Work out the finished part from the listing and answer in its coordinate system (mm). A direction names the side the tool comes from. Give positions to 0.01 mm unless a question says otherwise; leave off trailing zeros. Loops run counter-clockwise (first coordinate to the right, second up) from the corner with the lowest first, then second, coordinate; pieces in that order, holes last. Notation, with made-up numbers: (55, 64) - (69, 64) arc R13 ccw to (69, 89) - close; hole circle Ø3 at (-4, 0). An arc over 180 degrees is marked (long way). One line per item, written item: value.
from build123d import *

# Parameters (mm, degrees)
SKETCH1_W           = 25.4
SKETCH1_H           = 50.8
SKETCH1_W_2         = 19.05
SKETCH1_H_2         = 44.45
BOSS_EXTRUDE1_DEPTH = 736.6
SKETCH4_R           = 3.175
CUT_EXTRUDE1_DEPTH  = 3.175


with BuildPart() as part:
    # Sketch1 → Boss-Extrude1 (new body)
    with BuildSketch(Plane.XY):
        with Locations((12.7, 25.4)):
            Rectangle(SKETCH1_W, SKETCH1_H)
        with Locations((12.7, 25.4)):
            Rectangle(SKETCH1_W_2, SKETCH1_H_2, mode=Mode.SUBTRACT)
    extrude(amount=BOSS_EXTRUDE1_DEPTH)

    # Sketch4 → Cut-Extrude1 (cut)
    with BuildSketch(Plane.XZ):
        with Locations((12.7, 710.541764528)):
            Circle(SKETCH4_R)
        with Locations((12.7, 725.17)):
            Circle(SKETCH4_R)
        with Locations((12.7, 11.43)):
            Circle(SKETCH4_R)
        with Locations((12.7, 26.058235472)):
            Circle(SKETCH4_R)
    extrude(amount=-CUT_EXTRUDE1_DEPTH, mode=Mode.SUBTRACT)


solid = part.part
1. For faces 1 (the flat face through (13, 50.8, 363)), 2 (the flat face through (3.175, 25, 363)), determine the directions among +Z, -Z, +X, -X, +Y, -Y from which every point of the face is accessible in a straight line to the end or side of a thin tool.
Output:
face 1: +Z, -Z, +X, -X, +Y
face 2: +Z, -Z
2. Section A-A (z = 599) is taken. Write down the section's boundary in (x, y) (3 decimals).
Output:
outline: (0, 0) - (25.4, 0) - (25.4, 50.8) - (0, 50.8) - close; hole (3.175, 3.175) - (22.225, 3.175) - (22.225, 47.625) - (3.175, 47.625) - close
3. Flat-ended cylindrical pins translate along their axes: pin 1 Ø10 at (x, y) = (4.5, 21.5) entering from -Z; pin 2 Ø4 at (x, y) = (19, 15.5) entering from -Z; pin 3 Ø5.5 at (x, z) = (12.7, 11.43) entering from -Y (3 decimals). Find the tip coordinate at first contact, or state that the pin passes through.
Output:
pin 1: stops at z = 0
pin 2: passes through
pin 3: stops at y = 47.625
4. Find the intervals of material crossed by line 1 along Z through (x, y) = (12.7, 1.4) (3 decimals); line 2 along X through (y, z) = (8, 258) (3 decimals); line 3 along Y through (x, z) = (10.75, 615.5) (3 decimals), in increasing order.
Output:
line 1: z = 0 to 8.255, 14.605 to 22.883, 29.233 to 707.367, 713.717 to 721.995, 728.345 to 736.6
line 2: x = 0 to 3.175, 22.225 to 25.4
line 3: y = 0 to 3.175, 47.625 to 50.8
5. Section B-B (y = 16.5) is taken. Write down the section's boundary in (x, z) (3 decimals).
Output:
outline: (0, 0) - (3.175, 0) - (3.175, 736.6) - (0, 736.6) - close; (22.225, 0) - (25.4, 0) - (25.4, 736.6) - (22.225, 736.6) - close
6. The mould has two halves that part along Y. Classify faces 3 (the flat face through (2, 24, 736.6)), 4 (the flat face through (13, 0, 363)), 5 (the flat face through (13, 3.175, 363)), 6 (the flat face through (13, 47.625, 363)): released by +Y, released by -Y, zero draft, split by the parting line, or undercut.
Output:
face 3: zero draft
face 4: released by -Y
face 5: undercut
face 6: undercut
